Read the model definition and answer for the solid it produces. Units are mm, in the model's axes. Face numbers are marked on the shaded views. A direction names the side the tool comes from. Round coordinates to 2 decimals unless told otherwise and drop trailing zeros. Order: outer loops, then holes, each group sorted by start corner. A loop starts at its lowest first (then second) coordinate and runs counter-clockwise, first axis right, second up. Notation, with made-up numbers: (89.5, 1.5) - (136.5, 1.5) arc R30 ccw to (136.5, 24.5) - close; hole circle Ø2 at (68.5, -32.75). An arc over 180 degrees is marked (long way). Put each result on its own line as item: value. Start each with the question number.
Q1. For a pull along X with two mould halves and no side action, classify the marked faces 1, 2 and 3 as pulls with the +X half, pulls with the -X half, needs draft (parallel to the pull), parting line crosses it, or undercut.
Q2. Each of these flat-tipped pins is pushed along its axis until it touches: pin 1 Ø1.5 at (y, z) = (6.5, 48) entering from -X; pin 2 Ø8 at (x, y) = (-45, 8) entering from -Z; pin 3 Ø5.5 at (x, z) = (0, 0) entering from +Y. Where does it stop, or does it pass through?
Q3. Find the intervals of material crossed by line 1 along Y through (x, z) = (63.5, 2); line 2 along Y through (x, z) = (-6.5, -53.5); line 3 along Z through (x, y) = (25, 22), in increasing order. Write a range as from..to.
Q4. Which of the six approach directions +Z, -Z, +X, -X, +Y, -Y give full straight-line access (tool end or side, diameter ignored) to the marked faces 4, 5, 6 and 7?
Q5. Section D-D on x = 19 is taken. Give the vertices of the cut face in (y, z), then the cut area to 3 significant figures.
Q6. Section C-C on y = 8 is taken. Give the vertices of the cut face in (x, z).
Q7. Section B-B on x = 0 is taken. Give the vertices of the cut face in (y, z), then the cut area to 3 significant figures.
Q8. Section A-A on y = 31.5 is taken. Give the vertices of the cut face in (x, z), then the cut area to 3 significant figures.
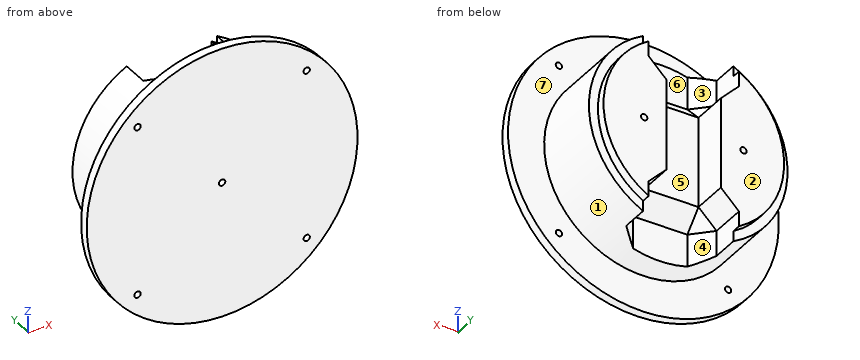
from build123d import *

# Parameters (mm, degrees)
SKETCH1_R                           = 55
BOSS_EXTRUDE1_DEPTH                 = 40
SKETCH2_R                           = 75
BOSS_EXTRUDE2_DEPTH                 = 5
SKETCH6_R                           = 50
BOSS_EXTRUDE3_DEPTH                 = 5
F_3_5_3_5_DIAMETER_HOLE1_D          = 3.5
F_3_5_3_5_DIAMETER_HOLE1_DEPTH      = 10
F_3_5_3_5_DIAMETER_HOLE1_TIP        = 1.051506083
SKETCH7_W                           = 50
SKETCH7_H                           = 60
CUT_EXTRUDE1_DEPTH                  = 30
CHAMFER1_SIZE                       = 10
SKETCH8_W                           = 30
SKETCH8_H                           = 50
CUT_EXTRUDE2_DEPTH                  = 20
F_3_5_3_5_DIAMETER_HOLE2_AT_2_COUNT = 2
F_3_5_3_5_DIAMETER_HOLE2_AT_2_PITCH = 66.25
F_3_5_3_5_DIAMETER_HOLE2_AT_3_COUNT = 2
F_3_5_3_5_DIAMETER_HOLE2_AT_3_PITCH = 66.25
F_3_5_3_5_DIAMETER_HOLE2_AT_4_COUNT = 2
F_3_5_3_5_DIAMETER_HOLE2_AT_4_PITCH = 66.25
F_3_5_3_5_DIAMETER_HOLE2_AT_5_COUNT = 2
F_3_5_3_5_DIAMETER_HOLE2_AT_5_PITCH = 66.25


with BuildPart() as part:
    # Sketch1 → Boss-Extrude1 (new body)
    with BuildSketch(Plane(origin=(0, 0, 0), x_dir=(1, 0, 0), z_dir=(0, 1, 0))):
        with Locations(Location((0, 0, 0), (0, 0, 270))):
            Circle(SKETCH1_R)
    extrude(amount=BOSS_EXTRUDE1_DEPTH)

    # Sketch2 → Boss-Extrude2 (add)
    with BuildSketch(Plane.XZ):
        with Locations(Location((0, 0, 0), (0, 0, 270))):
            Circle(SKETCH2_R)
    extrude(amount=BOSS_EXTRUDE2_DEPTH)

    # Sketch6 → Boss-Extrude3 (add)
    with BuildSketch(Plane(origin=(0, 40, 0), x_dir=(1, 0, 0), z_dir=(0, 1, 0))):
        with Locations(Location((0, 0, 0), (0, 0, 270))):
            Circle(SKETCH6_R)
    extrude(amount=BOSS_EXTRUDE3_DEPTH)

    # Ø3.5 (3.5) Diameter Hole1
    with Locations(Plane(origin=(-12.746034072, 45, -7.868896946), x_dir=(1, 0, 0), z_dir=(0, 1, 0))):
        with Locations((-14.753965928, -7.868896946), (40.246034072, -7.868896946)):
            Hole(F_3_5_3_5_DIAMETER_HOLE1_D / 2, depth=F_3_5_3_5_DIAMETER_HOLE1_DEPTH)
            with Locations((0, 0, -(F_3_5_3_5_DIAMETER_HOLE1_DEPTH + F_3_5_3_5_DIAMETER_HOLE1_TIP / 2))):  # 118° drill point
                Cone(0, F_3_5_3_5_DIAMETER_HOLE1_D / 2, F_3_5_3_5_DIAMETER_HOLE1_TIP, mode=Mode.SUBTRACT)

    # Sketch7 → Cut-Extrude1 (cut)
    with BuildSketch(Plane(origin=(0, 45, 0), x_dir=(1, 0, 0), z_dir=(0, 1, 0))):
        with Locations((0, 55)):
            Rectangle(SKETCH7_W, SKETCH7_H)
        with Locations((0, -55)):
            Rectangle(SKETCH7_W, SKETCH7_H)
    extrude(amount=-CUT_EXTRUDE1_DEPTH, mode=Mode.SUBTRACT)

    # Chamfer1
    chamfer1_edges = [part.edges().sort_by_distance(p)[0] for p in [
        (25, 15, -36.994897428),
        (-25, 15, -36.994897428),
        (-25, 30, -25),
        (0, 15, -25),
        (25, 30, -25),
        (25, 15, 36.994897428),
        (25, 30, 25),
        (-25, 15, 36.994897428),
        (0, 15, 25),
        (-25, 30, 25),
    ]]
    chamfer(chamfer1_edges, length=CHAMFER1_SIZE)

    # Sketch8 → Cut-Extrude2 (cut)
    with BuildSketch(Plane(origin=(0, 45, 0), x_dir=(1, 0, 0), z_dir=(0, 1, 0))):
        Rectangle(SKETCH8_W, SKETCH8_H)
    extrude(amount=-CUT_EXTRUDE2_DEPTH, mode=Mode.SUBTRACT)

    # Sketch9 → Ø3.5 (3.5) Diameter Hole2 (revolve, cut)
    with BuildSketch(Plane(origin=(0, 0, 0), x_dir=(0, 0, 1), z_dir=(1, 0, 0))):
        Polygon((0, 0), (0, 11.051506083), (1.75, 10), (1.75, 0), align=None)
    f_3_5_3_5_diameter_hole2 = revolve(axis=Axis((0, 6.35, 0), (0, -1, 0)), mode=Mode.SUBTRACT)

    # Ø3.5 (3.5) Diameter Hole2 at 2: Ø3.5 (3.5) Diameter Hole2 ×2
    with Locations(*[Vector(0.7071067811865477, 0, 0.7071067811865475) * (i * F_3_5_3_5_DIAMETER_HOLE2_AT_2_PITCH) for i in range(1, F_3_5_3_5_DIAMETER_HOLE2_AT_2_COUNT)]):
        add(f_3_5_3_5_diameter_hole2, mode=Mode.SUBTRACT)

    # Ø3.5 (3.5) Diameter Hole2 at 3: Ø3.5 (3.5) Diameter Hole2 ×2
    with Locations(*[Vector(-0.7071067811865478, 0, -0.7071067811865474) * (i * F_3_5_3_5_DIAMETER_HOLE2_AT_3_PITCH) for i in range(1, F_3_5_3_5_DIAMETER_HOLE2_AT_3_COUNT)]):
        add(f_3_5_3_5_diameter_hole2, mode=Mode.SUBTRACT)

    # Ø3.5 (3.5) Diameter Hole2 at 4: Ø3.5 (3.5) Diameter Hole2 ×2
    with Locations(*[Vector(-0.7071067811865476, 0, 0.7071067811865476) * (i * F_3_5_3_5_DIAMETER_HOLE2_AT_4_PITCH) for i in range(1, F_3_5_3_5_DIAMETER_HOLE2_AT_4_COUNT)]):
        add(f_3_5_3_5_diameter_hole2, mode=Mode.SUBTRACT)

    # Ø3.5 (3.5) Diameter Hole2 at 5: Ø3.5 (3.5) Diameter Hole2 ×2
    with Locations(*[Vector(0.7071067811865476, 0, -0.7071067811865476) * (i * F_3_5_3_5_DIAMETER_HOLE2_AT_5_PITCH) for i in range(1, F_3_5_3_5_DIAMETER_HOLE2_AT_5_COUNT)]):
        add(f_3_5_3_5_diameter_hole2, mode=Mode.SUBTRACT)


solid = part.part
Findings:
1. face 1: parting line crosses it
1. face 2: needs draft
1. face 3: undercut
2. pin 1: x = -28.15
2. pin 2: z = -36.66
2. pin 3: y = 25
3. line 1: -5..0
3. line 2: -5..15
3. line 3: -48.99..48.99
4. face 4: -Z, +Y
4. face 5: +Z, -Z, +Y
4. face 6: +Z, +Y
4. face 7: +Y
5. outline: (-5, -72.55) - (0, -72.55) - (0, -51.61) - (19, -51.61) - (19, -35) - (25, -29) - (45, -29) - (45, 29) - (25, 29) - (19, 35) - (19, 51.61) - (0, 51.61) - (0, 72.55) - (-5, 72.55) - close
5. area: 4,230 mm2
6. outline: circle Ø110 at (0, 0)
7. outline: (-5, -75) - (0, -75) - (0, -55) - (15, -55) - (15, -35) - (25, -25) - (25, 25) - (15, 35) - (15, 55) - (0, 55) - (0, 75) - (-5, 75) - (-5, 1.75) - (0, 1.75) - (0, -1.75) - (-5, -1.75) - close
7. area: 2,980 mm2
8. outline: (-25, -48.99) - (-25, -35) - (-15, -25) - (-15, 25) - (-25, 35) - (-25, 48.99) arc R55 ccw to start; (15, -25) - (25, -35) - (25, -48.99) arc R55 ccw to (25, 48.99) - (25, 35) - (15, 25) - close
8. area: 5,400 mm2
